Source: CAD feature listing. Evaluate the final solid. Frame: model axes, mm. A direction names the side the tool comes from. Give positions to 0.01 mm unless a question says otherwise; leave off trailing zeros. Loops run counter-clockwise (first coordinate to the right, second up) from the corner with the lowest first, then second, coordinate; pieces in that order, holes last. Notation, with made-up numbers: (-29.75, 10) - (29.25, 10) arc R12 cw to (29.25, 30) - close; hole circle Ø10 at (-24.5, 86). An arc over 180 degrees is marked (long way). Put each result on its own line as item: value.
```python
from build123d import *

# Parameters (mm, degrees)
SKETCH1_W               = 20
SKETCH1_H               = 40
BOSS_EXTRUDE1_DEPTH     = 11
SKETCH2_W               = 18
SKETCH2_H               = 9
CUT_EXTRUDE1_DEPTH      = 39
SKETCH3_W               = 10
SKETCH3_H               = 5
CUT_EXTRUDE2_DEPTH      = 6
CUT_EXTRUDE2_DEPTH_BACK = 4


with BuildPart() as part:
    # Sketch1 → Boss-Extrude1 (new body)
    with BuildSketch(Plane.XY):
        with Locations((-15.909713685, 10.402437659)):
            Rectangle(SKETCH1_W, SKETCH1_H)
    extrude(amount=BOSS_EXTRUDE1_DEPTH)

    # Sketch2 → Cut-Extrude1 (cut)
    with BuildSketch(Plane(origin=(0, 30.402437659, 0), x_dir=(1, 0, 0), z_dir=(0, 1, 0))):
        with Locations((-15.909713685, -5.5)):
            Rectangle(SKETCH2_W, SKETCH2_H)
    extrude(amount=-CUT_EXTRUDE1_DEPTH, mode=Mode.SUBTRACT)

    # Sketch3 → Cut-Extrude2 (cut, two sides)
    with BuildSketch(Plane.XY.offset(11)) as cut_extrude2_sk:
        with Locations((-15.909713685, 15.902437659)):
            Rectangle(SKETCH3_W, SKETCH3_H)
        with Locations((-15.909713685, 0.902437659)):
            Rectangle(SKETCH3_W, SKETCH3_H)
    extrude(amount=CUT_EXTRUDE2_DEPTH, mode=Mode.SUBTRACT)
    extrude(cut_extrude2_sk.sketch, amount=-CUT_EXTRUDE2_DEPTH_BACK, mode=Mode.SUBTRACT)


solid = part.part
```
1) Section query D-D, the plane y = 2. Output: boundary loops of the cut face in (x, z).
Check result:
outline: (-25.91, 0) - (-5.91, 0) - (-5.91, 11) - (-10.91, 11) - (-10.91, 10) - (-6.91, 10) - (-6.91, 1) - (-24.91, 1) - (-24.91, 10) - (-20.91, 10) - (-20.91, 11) - (-25.91, 11) - close
2) Section query C-C, the plane z = 2.5. Output: boundary loops of the cut face in (x, y), plus the area to 3 significant figures.
Check result:
outline: (-25.91, -9.6) - (-5.91, -9.6) - (-5.91, 30.4) - (-6.91, 30.4) - (-6.91, -8.6) - (-24.91, -8.6) - (-24.91, 30.4) - (-25.91, 30.4) - close
area: 98.0 mm²
3) Section query A-A, the plane y = 22. Output: boundary loops of the cut face in (x, z), plus the area to 3 significant figures.
Check result:
outline: (-25.91, 0) - (-5.91, 0) - (-5.91, 11) - (-25.91, 11) - close; hole (-24.91, 1) - (-6.91, 1) - (-6.91, 10) - (-24.91, 10) - close
area: 58.0 mm²
4) Access query for faces 5 (the flat face through (-16, 3.402, 10.5)), 6 (the flat face through (-16, 11, 10)), 7 (the flat face through (-16, 11, 0)). Directions: +Z, -Z, +X, -X, +Y, -Y. A direction counts if a zero-diameter tool reaches every point of the face in a straight line with its end or side. Return the directions, or none.
Check result:
face 5: +Z
face 6: +Y
face 7: -Z, +X, -X, +Y, -Y
5) Mould query, pull axis X, two halves, no side actions, for faces 1 (the flat face through (-16, 30.402, 0.6)), 2 (the flat face through (-25.91, 10, 5)), 3 (the flat face through (-16, -8.598, 5)), 4 (the flat face through (-6.91, 11, 6)). Classes: pulls with the +X half, pulls with the -X half, needs draft (parallel to the pull), parting line crosses it, or undercut.
Check result:
face 1: needs draft
face 2: pulls with the -X half
face 3: undercut
face 4: undercut
6) Material intervals for line 1 along X through (y, z) = (21, 3); line 2 along Z through (x, y) = (-18.5, 20.5); line 3 along Y through (x, z) = (-12.25, 10.25), sorted ascending. Write a range as [from, to].
Check result:
line 1: [-25.91, -24.91], [-6.91, -5.91]
line 2: [0, 1], [10, 11]
line 3: [-9.6, -1.6], [3.4, 13.4], [18.4, 30.4]
7) Section query B-B, the plane x = -14. Output: boundary loops of the cut face in (y, z).
Check result:
outline: (-9.6, 0) - (30.4, 0) - (30.4, 1) - (-8.6, 1) - (-8.6, 10) - (-1.6, 10) - (-1.6, 11) - (-9.6, 11) - close; (3.4, 10) - (13.4, 10) - (13.4, 11) - (3.4, 11) - close; (18.4, 10) - (30.4, 10) - (30.4, 11) - (18.4, 11) - close
8) Pin query (flat end, axial travel): P1, Ø1, axis at x = -10, z = 5, coming from the +Y side. Return the tip coordinate at first contact, or that it passes through.
Check result:
P1: y = -8.6
